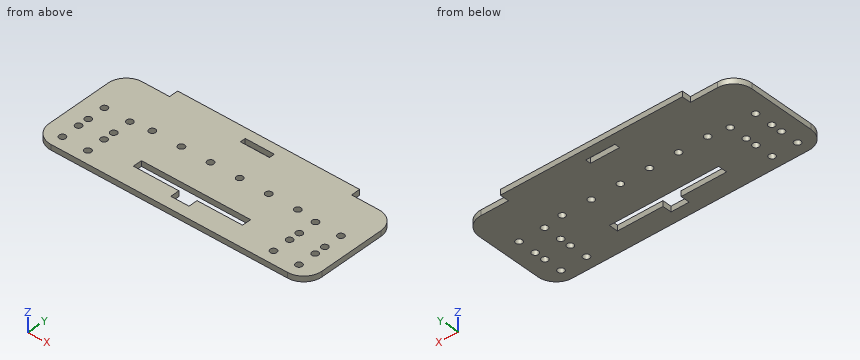
```python
from build123d import *

# Parameters (mm, degrees)
BOSS_EXTRUDE1_DEPTH = 3
SKETCH2_R           = 1.8
SKETCH2_W           = 60
SKETCH2_H           = 5
SKETCH2_W_2         = 16
SKETCH2_H_2         = 3
CUT_EXTRUDE1_DEPTH  = 5
SKETCH3_W           = 10
SKETCH3_H           = 5
CUT_EXTRUDE2_DEPTH  = 10


with BuildPart() as part:
    # Sketch1 → Boss-Extrude1 (new body)
    with BuildSketch(Plane.XY):
        with BuildLine():
            Line((-65, 28.25), (-50, 28.25))
            Line((-50, 28.25), (-50, 33.25))
            Line((-50, 33.25), (50, 33.25))
            Line((50, 33.25), (50, 28.25))
            Line((50, 28.25), (65, 28.25))
            ThreePointArc((65, 28.25), (72.071067812, 25.321067812), (75, 18.25))
            Line((75, 18.25), (75, -18.25))
            ThreePointArc((75, -18.25), (72.071067812, -25.321067812), (65, -28.25))
            Line((65, -28.25), (-65, -28.25))
            ThreePointArc((-65, -28.25), (-72.071067812, -25.321067812), (-75, -18.25))
            Line((-75, -18.25), (-75, 18.25))
            ThreePointArc((-75, 18.25), (-72.071067812, 25.321067812), (-65, 28.25))
        make_face()
    extrude(amount=BOSS_EXTRUDE1_DEPTH)

    # Sketch2 → Cut-Extrude1 (cut)
    with BuildSketch(Plane.XY.offset(3)):
        with Locations((-65, -21.25)):
            Circle(SKETCH2_R)
        with Locations((-65, -11.25)):
            Circle(SKETCH2_R)
        with Locations((-65, -5.25)):
            Circle(SKETCH2_R)
        with Locations((-51, -5.25)):
            Circle(SKETCH2_R)
        with Locations((-51, -11.25)):
            Circle(SKETCH2_R)
        with Locations((-51, -21.25)):
            Circle(SKETCH2_R)
        with Locations((51, -5.25)):
            Circle(SKETCH2_R)
        with Locations((51, -11.25)):
            Circle(SKETCH2_R)
        with Locations((51, -21.25)):
            Circle(SKETCH2_R)
        with Locations((65, -21.25)):
            Circle(SKETCH2_R)
        with Locations((65, -11.25)):
            Circle(SKETCH2_R)
        with Locations((65, -5.25)):
            Circle(SKETCH2_R)
        with Locations((-65, 4.75)):
            Circle(SKETCH2_R)
        with Locations((-51, 4.75)):
            Circle(SKETCH2_R)
        with Locations((65, 4.75)):
            Circle(SKETCH2_R)
        with Locations((51, 4.75)):
            Circle(SKETCH2_R)
        with Locations((24, 6.25)):
            Circle(SKETCH2_R)
        with Locations((40, 6.25)):
            Circle(SKETCH2_R)
        with Locations((-40, 6.25)):
            Circle(SKETCH2_R)
        with Locations((-24, 6.25)):
            Circle(SKETCH2_R)
        with Locations((8, 6.25)):
            Circle(SKETCH2_R)
        with Locations((-8, 6.25)):
            Circle(SKETCH2_R)
        with Locations((0, -14.25)):
            Rectangle(SKETCH2_W, SKETCH2_H)
        with Locations((0, 26.25)):
            Rectangle(SKETCH2_W_2, SKETCH2_H_2)
    extrude(amount=-CUT_EXTRUDE1_DEPTH, mode=Mode.SUBTRACT)

    # Sketch3 → Cut-Extrude2 (cut)
    with BuildSketch(Plane.XY.offset(3)):
        with Locations((0, -19.25)):
            Rectangle(SKETCH3_W, SKETCH3_H)
    extrude(amount=-CUT_EXTRUDE2_DEPTH, mode=Mode.SUBTRACT)


solid = part.part
```
Here's how the part is built. I have some questions about the finished solid (model axes, mm). Round coordinates to 2 decimals unless told otherwise and drop trailing zeros. Loops run counter-clockwise (first coordinate to the right, second up) from the corner with the lowest first, then second, coordinate; pieces in that order, holes last. Notation, with made-up numbers: (39.5, -34.75) -> (95.5, -34.75) arc R11 cw to (95.5, -13.75) -> close; hole circle Ø5 at (19, 41). An arc over 180 degrees is marked (long way). Answer as CSV lines item,"result".
1. If we section it at C-C on x = 2: Please give me the cut outline in (y, z), plus the area to 4 significant figures.
Final values:
outline,"(-28.25, 0) -> (-21.75, 0) -> (-21.75, 3) -> (-28.25, 3) -> close; (-11.75, 0) -> (24.75, 0) -> (24.75, 3) -> (-11.75, 3) -> close; (27.75, 0) -> (33.25, 0) -> (33.25, 3) -> (27.75, 3) -> close"
area,"145.5 mm^2"
2. If we section it at D-D on z = 1.25: Count the separate pieces of the cut face and the enclosed holes in it, plus the area to 3 significant figures.
Final values:
separate pieces,"1"
enclosed holes,"24"
area,"8,270 mm^2"
3. If we section it at A-A on y = -5.25: Please give me the cut outline in (x, z), plus the area to 3 significant figures.
Final values:
outline,"(-75, 0) -> (-66.8, 0) -> (-66.8, 3) -> (-75, 3) -> close; (-63.2, 0) -> (-52.8, 0) -> (-52.8, 3) -> (-63.2, 3) -> close; (-49.2, 0) -> (49.2, 0) -> (49.2, 3) -> (-49.2, 3) -> close; (52.8, 0) -> (63.2, 0) -> (63.2, 3) -> (52.8, 3) -> close; (66.8, 0) -> (75, 0) -> (75, 3) -> (66.8, 3) -> close"
area,"407 mm^2"
4. If we section it at B-B on x = 24: Please give me the cut outline in (y, z).
Final values:
outline,"(-28.25, 0) -> (-16.75, 0) -> (-16.75, 3) -> (-28.25, 3) -> close; (-11.75, 0) -> (4.45, 0) -> (4.45, 3) -> (-11.75, 3) -> close; (8.05, 0) -> (33.25, 0) -> (33.25, 3) -> (8.05, 3) -> close"
5. If I drill on L1, parallel to X at y = -5, z = 1.75; L2, parallel to Y at x = 51, z = 1.55; L3, parallel to Y at x = -26, z = 1.8, over which ranges is the centre line in solid material (lowest first)?
Final values:
L1,"x = -75 to -66.78, -63.22 to -52.78, -49.22 to 49.22, 52.78 to 63.22, 66.78 to 75"
L2,"y = -28.25 to -23.05, -19.45 to -13.05, -9.45 to -7.05, -3.45 to 2.95, 6.55 to 28.25"
L3,"y = -28.25 to -16.75, -11.75 to 33.25"
6. For pin 1 (0.9 mm diameter, centred on x = -55.5, z = 1.5, fed in from +Y); pin 2 (1.5 mm diameter, centred on y = 30, z = 2, fed in from -X); pin 3 (0.9 mm diameter, centred on y = 31.5, z = 1, fed in from +X), each with a flat end and sliding along its axis, tell me the tip position at first contact or that it passes through.
Final values:
pin 1,"stops at y = 28.25"
pin 2,"stops at x = -50"
pin 3,"stops at x = 50"
